```python
from build123d import *

# Parameters (mm, degrees)
F1_DEPTH = 25.4
F2_W     = 18.447345
F2_H     = 17.589332
F3_DEPTH = 25.4
F4_W     = 16.731317
F4_H     = 16.731312
F5_DEPTH = 25.4
F6_W     = 18.750374
F6_H     = 18.53587
F7_DEPTH = 25.4


with BuildPart() as f1:
    # F0 (on Front) → F1 (new body)
    with BuildSketch(Plane.XZ):
        Polygon((-25.4, 0), (0, 0), (0, 25.4), (-1.806476, 25.4), (-25.4, 25.4), align=None)
    extrude(amount=F1_DEPTH)

    # F2 (on face) → F3 (cut)
    with BuildSketch(Plane.XZ.offset(25.4)):
        with Locations((-12.762988, 12.870242)):
            Rectangle(F2_W, F2_H)
    extrude(amount=-F3_DEPTH, mode=Mode.SUBTRACT)

    # F4 (on face) → F5 (cut)
    with BuildSketch(Plane.YZ):
        with Locations((-12.762989, 12.870242)):
            Rectangle(F4_W, F4_H)
    extrude(amount=-F5_DEPTH, mode=Mode.SUBTRACT)

    # F6 (on face) → F7 (cut)
    with BuildSketch(Plane.XY.offset(25.4)):
        with Locations((-12.7, -12.7)):
            Rectangle(F6_W, F6_H)
    extrude(amount=-F7_DEPTH, mode=Mode.SUBTRACT)


solid = f1.part
```
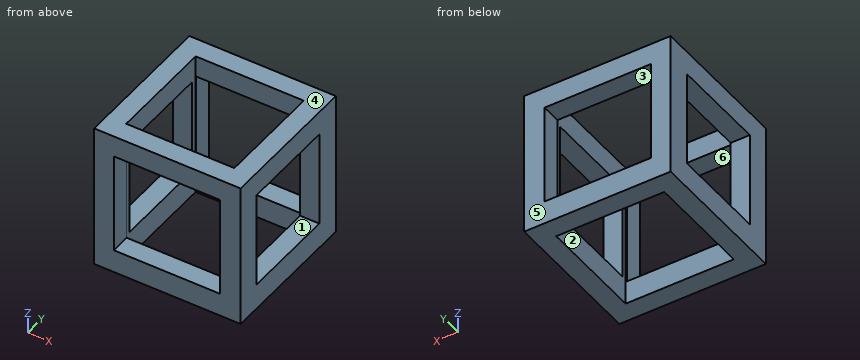
Read the model definition and answer for the solid it produces. Units are mm, in the model's axes. Face numbers are marked on the shaded views. A direction names the side the tool comes from. Coordinates: 2 decimals unless noted, no trailing zeros. Write each loop counter-clockwise with the first axis right and the second up, starting at its lowest first coordinate (ties: lowest second). Pieces come first, ordered by that corner, then holes. Notation, with made-up numbers: (-10, 67.25) -> (43, 67.25) arc R21 ccw to (43, 84.25) -> close; hole circle Ø5 at (30.25, -19.75). An arc over 180 degrees is marked (long way). Write item = value, one per line.
(1) Section A-A on x = -10.25 is taken. Write down the section's boundary in (y, z), plus the area to 3 significant figures.
From the geometry:
outline = (-25.4, 0) -> (-21.97, 0) -> (-21.97, 4.08) -> (-25.4, 4.08) -> close; (-25.4, 21.66) -> (-21.97, 21.66) -> (-21.97, 25.4) -> (-25.4, 25.4) -> close; (-3.43, 0) -> (0, 0) -> (0, 4.08) -> (-3.43, 4.08) -> close; (-3.43, 21.66) -> (0, 21.66) -> (0, 25.4) -> (-3.43, 25.4) -> close
area = 53.6 mm2
(2) Section C-C on y = -14.25 is taken. Write down the section's boundary in (x, z), plus the area to 3 significant figures.
From the geometry:
outline = (-25.4, 0) -> (-22.08, 0) -> (-22.08, 4.5) -> (-25.4, 4.5) -> close; (-25.4, 21.24) -> (-22.08, 21.24) -> (-22.08, 25.4) -> (-25.4, 25.4) -> close; (-3.32, 0) -> (0, 0) -> (0, 4.5) -> (-3.32, 4.5) -> close; (-3.32, 21.24) -> (0, 21.24) -> (0, 25.4) -> (-3.32, 25.4) -> close
area = 57.6 mm2
(3) Straight lines are drawn through the part: L1, parallel to X at y = -21.75, z = 6.25; L2, parallel to X at y = -1.25, z = 6.25; L3, parallel to Z at x = -13.25, y = -23. For each, find the intervals that lie inside material, in ascending order. Write a range as from..to.
From the geometry:
L1 = -25.4..-22.08, -3.32..0
L2 = -25.4..-21.99, -3.54..0
L3 = 0..4.08, 21.66..25.4
(4) Which of the six approach directions +Z, -Z, +X, -X, +Y, -Y give full straight-line access (tool end or side, diameter ignored) to the marked faces 1, 2 and 3?
From the geometry:
face_1 = +X, -X
face_2 = +Z, -Z
face_3 = +Y, -Y
(5) For a pull along Z with two mould halves and no side action, classify the marked faces 4, 5 and 6 as +Z half, -Z half, draft (parallel to the pull), parting line (faces both ways), or undercut.
From the geometry:
face_4 = +Z half
face_5 = draft
face_6 = undercut
(6) Section D-D on z = 23 is taken. Write down the section's boundary in (x, y).
From the geometry:
outline = (-25.4, -25.4) -> (0, -25.4) -> (0, 0) -> (-25.4, 0) -> close; hole (-22.08, -21.97) -> (-3.32, -21.97) -> (-3.32, -3.43) -> (-22.08, -3.43) -> close
(7) Section B-B on z = 20.25 is taken. Write down the section's boundary in (x, y).
From the geometry:
outline = (-25.4, -25.4) -> (-21.99, -25.4) -> (-21.99, -21.97) -> (-22.08, -21.97) -> (-22.08, -21.13) -> (-25.4, -21.13) -> close; (-25.4, -4.4) -> (-22.08, -4.4) -> (-22.08, -3.43) -> (-21.99, -3.43) -> (-21.99, 0) -> (-25.4, 0) -> close; (-3.54, -25.4) -> (0, -25.4) -> (0, -21.13) -> (-3.32, -21.13) -> (-3.32, -21.97) -> (-3.54, -21.97) -> close; (-3.54, -3.43) -> (-3.32, -3.43) -> (-3.32, -4.4) -> (0, -4.4) -> (0, 0) -> (-3.54, 0) -> close
